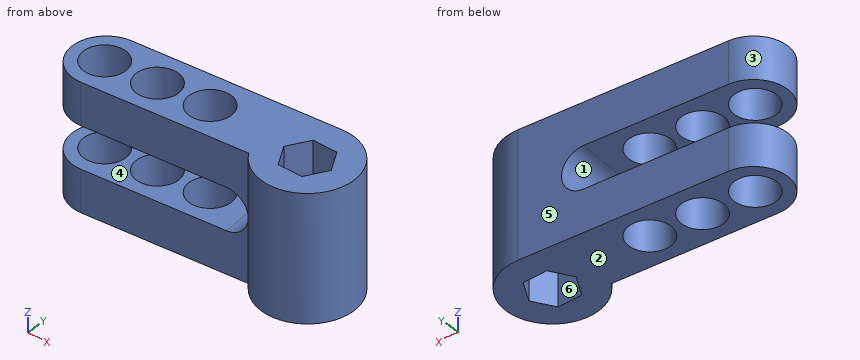
from build123d import *

# Parameters (mm, degrees)
BOSS_EXTRUDE1_DEPTH = 30
CUT_EXTRUDE1_DEPTH  = 23.916854849
SKETCH3_R           = 5
CUT_EXTRUDE2_DEPTH  = 31


with BuildPart() as part:
    # Sketch1 → Boss-Extrude1 (new body)
    with BuildSketch(Plane.XY):
        with BuildLine():
            Line((23.159950064, 11.160474583), (-24.578582707, 6.983894152))
            ThreePointArc((-24.578582707, 6.983894152), (-31.85089435, -1.682909374), (-23.184090823, -8.955221017))
            Line((-23.184090823, -8.955221017), (14.793767169, -5.632588978))
            ThreePointArc((14.793767169, -5.632588978), (33.964469482, -4.702776608), (23.159950064, 11.160474583))
        make_face()
        Polygon((27.005414581, -4.797667096), (29.892165926, 0.202332904), (27.005414581, 5.202332904), (21.231911889, 5.202332904), (18.345160543, 0.202332904), (21.231911889, -4.797667096), align=None, mode=Mode.SUBTRACT)
    extrude(amount=BOSS_EXTRUDE1_DEPTH)

    # Sketch2 → Cut-Extrude1 (cut, through all)
    with BuildSketch(Plane(origin=(-0.793072196, 9.064856678, 0), x_dir=(0.996194698, 0.087155743, 0), z_dir=(-0.087155743, 0.996194698, 0))):
        with BuildLine():
            Line((-32.881194949, -10), (9.118805051, -10))
            ThreePointArc((9.118805051, -10), (14.118805051, -15), (9.118805051, -20))
            Line((9.118805051, -20), (-32.881194949, -20))
            Line((-32.881194949, -20), (-32.881194949, -10))
        make_face()
    extrude(amount=-CUT_EXTRUDE1_DEPTH, mode=Mode.SUBTRACT)

    # Sketch3 → Cut-Extrude2 (cut, through all)
    with BuildSketch(Plane.XY.offset(30)):
        with Locations((-24.243526624, -1.017350939)):
            Circle(SKETCH3_R)
        with Locations((-12.289190247, 0.028517974)):
            Circle(SKETCH3_R)
        with Locations((-0.33485387, 1.074386887)):
            Circle(SKETCH3_R)
    extrude(amount=-CUT_EXTRUDE2_DEPTH, mode=Mode.SUBTRACT)


solid = part.part
Geometry: final body of the model. Coordinates: model frame, mm. Face numbers are marked on the shaded views. A direction names the side the tool comes from. Round coordinates to 2 decimals unless told otherwise and drop trailing zeros. Loops run counter-clockwise (first coordinate to the right, second up) from the corner with the lowest first, then second, coordinate; pieces in that order, holes last. Notation, with made-up numbers: (40, 77.5) - (50, 77.5) arc R13 cw to (50, 98.5) - close; hole circle Ø9 at (-10, 77.25). An arc over 180 degrees is marked (long way). Write each question's results on one line, items separated by ' | '. Start each with the question number.
1) Cut plane C-C on y = 2.5. Count the separate pieces of the cut face and the enclosed holes in it, then the cut area to 3 significant figures.
2) Access query for the marked faces 5 and 6. Directions: +Z, -Z, +X, -X, +Y, -Y. A direction counts if a zero-diameter tool reaches every point of the face in a straight line with its end or side. Return the directions, or none.
3) Cut plane D-D on z = 21.5. Return loops of the section in (x, y), then the cut area to 3 significant figures.
4) Mould query, pull axis Z, two halves, no side actions, for the marked faces 1, 2, 3 and 4. Classes: released by +Z, released by -Z, zero draft, split by the parting line, or undercut.
5) Line query: probe 1 along Z at (x, y) = (6, -4); probe 2 along Y at (x, z) = (-3, 26.75); probe 3 along Z at (x, y) = (13, -0.25). Output: solid intervals per line, ascending. Write a range as [from, to].
6) First-contact query: P1, Ø6.5, axis at x = 24.5, z = 17.5, coming from the +Y side; P2, Ø1.5, axis at y = 2.5, z = 5, coming from the +X side; P3, Ø8, axis at y = 6.5, z = 24, coming from the -X side; P4, Ø5, axis at y = -2.5, z = 8, coming from the +X side. Flat tips, straight axial feed; report the tip coordinate or a pass-through.
7) Cut plane A-A on x = -20. Return loops of the section in (y, z), then the cut area to 3 significant figures.
8) Cut plane B-B on z = 18.5. Return loops of the section in (x, y).
Verdict:
1) separate pieces: 8 | enclosed holes: 0 | area: 765 mm2
2) face 5: +Z, -Z, -X, +Y | face 6: +Z, -Z
3) outline: (-24.58, 6.98) arc R8 ccw to (-23.18, -8.96) - (14.79, -5.63) arc R11 ccw (long way) to (23.16, 11.16) - close; hole circle Ø10 at (-24.24, -1.02); hole circle Ø10 at (-12.29, 0.03); hole circle Ø10 at (-0.33, 1.07); hole (18.35, 0.2) - (21.23, -4.8) - (27.01, -4.8) - (29.89, 0.2) - (27.01, 5.2) - (21.23, 5.2) - close | area: 777 mm2
4) face 1: undercut | face 2: released by -Z | face 3: zero draft | face 4: undercut
5) probe 1: z = [0, 10], [20, 30] | probe 2: y = [-7.19, -3.16], [5.3, 8.87] | probe 3: z = [0, 11.76], [18.24, 30]
6) P1: stops at y = 11.2 | P2: stops at x = 35.01 | P3: stops at x = -31.08 | P4: stops at x = 35.12
7) outline: (-8.68, 0) - (-3.66, 0) - (-3.66, 10) - (-8.68, 10) - close; (-8.68, 20) - (-3.66, 20) - (-3.66, 30) - (-8.68, 30) - close; (1.63, 0) - (7.38, 0) - (7.38, 10) - (1.63, 10) - close; (1.63, 20) - (7.38, 20) - (7.38, 30) - (1.63, 30) - close | area: 215 mm2
8) outline: (11.85, 10.17) - (13.24, -5.77) - (14.79, -5.63) arc R11 ccw (long way) to (23.16, 11.16) - close; hole (18.35, 0.2) - (21.23, -4.8) - (27.01, -4.8) - (29.89, 0.2) - (27.01, 5.2) - (21.23, 5.2) - close
